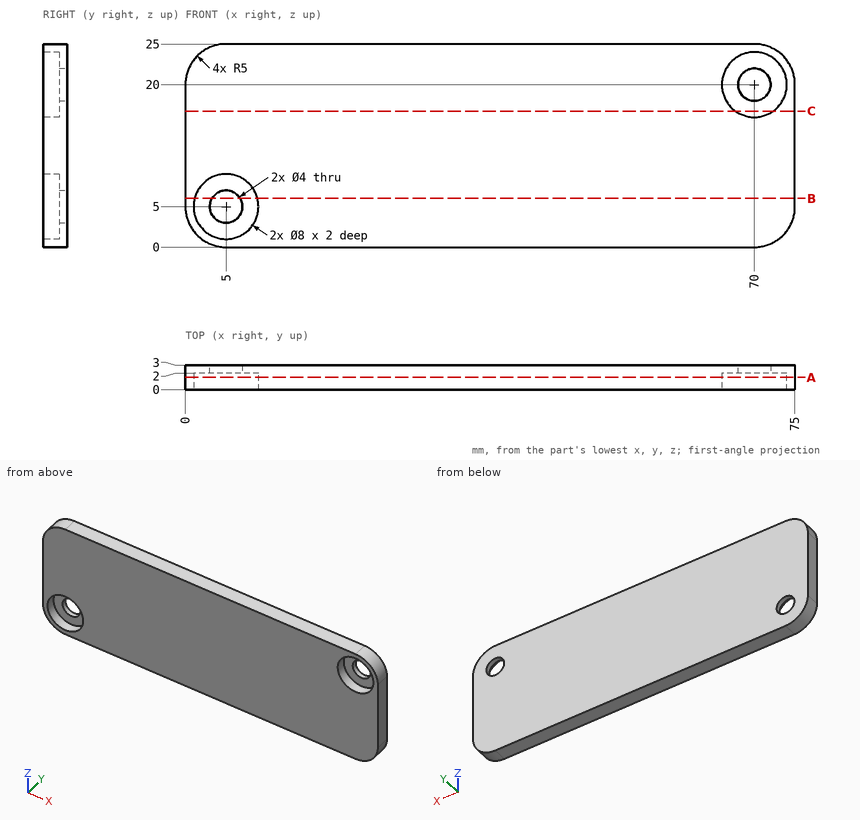
Check sheet for the drawn part. Datum: minimum x, y, z corner. Units: mm. Coordinates: 2 decimals unless noted, no trailing zeros. Order: outer loops, then holes, each group sorted by start corner. A loop starts at its lowest first (then second) coordinate and runs counter-clockwise, first axis right, second up. Notation, with made-up numbers: M 84.5,-7.75 L 123.5,-7.75 A36 cw 123.5,28.25 Z; hole C 61.25,13 d10. An arc over 180 degrees is marked long. One line per question, with ' | ' between items. Start each with the question number.
Item 1: Cross-section at C-C on z = 16.75. Enter the section's corners in (x, y).
Item 2: Gauge pin test, flat ends, axial feed: pin 1 (5 mm diameter, centred on x = 70, z = 20, fed in from -Y); pin 2 (2.5 mm diameter, centred on x = 5, z = 5, fed in from +Y). Record the tip position at first contact, or that the pin passes through.
Item 3: Cross-section at A-A on y = 1.5. Enter the section's corners in (x, z), then the cut area to 3 significant figures.
Item 4: Material ranges on L1, parallel to X at y = 1, z = 19.75; L2, parallel to Z at x = 71.5, y = 2.7; L3, parallel to X at y = 2.95, z = 23, recorded low to high. Write a range as [from, to].
Item 5: Cross-section at B-B on z = 6. Enter the section's corners in (x, y).
Findings:
1) outline: M 0,0 L 67.67,0 L 67.67,2 L 72.33,2 L 72.33,0 L 75,0 L 75,3 L 0,3 Z
2) pin 1: stops at y = 2 | pin 2: passes through
3) outline: M 0,5 A5 ccw 5,0 L 70,0 A5 ccw 75,5 L 75,20 A5 ccw 70,25 L 5,25 A5 ccw 0,20 Z; hole C 5,5 d8; hole C 70,20 d8 | area: 1,750 mm²
4) L1: x = [0, 66.01], [73.99, 75] | L2: z = [0.23, 18.68], [21.32, 24.77] | L3: x = [1, 74]
5) outline: M 0,0 L 1.13,0 L 1.13,2 L 3.27,2 L 3.27,3 L 0,3 Z; M 6.73,2 L 8.87,2 L 8.87,0 L 75,0 L 75,3 L 6.73,3 Z
